Source: CAD feature listing. Evaluate the final solid. Frame: model axes, mm. A direction names the side the tool comes from. Give positions to 0.01 mm unless a question says otherwise; leave off trailing zeros. Write each loop counter-clockwise with the first axis right and the second up, starting at its lowest first coordinate (ties: lowest second). Pieces come first, ordered by that corner, then holes. Notation, with made-up numbers: (61, 76) -> (69, 76) arc R33 ccw to (69, 108) -> close; hole circle Ø5 at (-15.75, 75). An arc over 180 degrees is marked (long way). Use one line per item in the form item = value. Start each with the question number.
(1) First-contact query: P1, Ø5, axis at x = 27, z = 207.5, coming from the -Y side; P2, Ø10, axis at x = 14.5, y = 35.5, coming from the -Z side; P3, Ø8, axis at y = 4.5, z = 180, coming from the -X side. Flat tips, straight axial feed; report the tip coordinate or a pass-through.
(2) Material intervals for line 1 along Y through (x, z) = (0, 8.2); line 2 along Z through (x, y) = (-4, -11); line 3 along Z through (x, y) = (49.5, -9.5), sorted ascending. Write a range as from..to.
(3) Set-up query: faces 1 (the face through (-39.017, 35.777, 144.998)), 2 (the face through (1, 1, 10)), 3 (the face through (45.723, 14.399, 317.255)). Return all of +Z, -Z, +X, -X, +Y, -Y with unobstructed straight access to the full face (end or side cutting, diameter ignored); none if empty.
(4) Cut plane B-B, the plane z = 95. Output: boundary loops of the cut face in (x, y), and give its area (3 significant figures).
from build123d import *

# Parameters (mm, degrees)
SKETCH1_R           = 52.936641772
BOSS_EXTRUDE1_DEPTH = 300
FILLET1_R           = 10
SKETCH2_R           = 47.936641772
BOSS_EXTRUDE2_DEPTH = 50
FILLET2_R           = 15
SKETCH3_R           = 43.922720163
CUT_EXTRUDE1_DEPTH  = 10
FILLET3_R           = 5
FILLET4_R           = 4


with BuildPart() as part:
    # Sketch1 → Boss-Extrude1 (new body)
    with BuildSketch(Plane.XY):
        Circle(SKETCH1_R)
    extrude(amount=BOSS_EXTRUDE1_DEPTH)

    # Fillet1
    fillet1_edges = [part.edges().sort_by_distance(p)[0] for p in [
        (-52.936641772, 0, 300),
    ]]
    fillet(fillet1_edges, radius=FILLET1_R)

    # Sketch2 → Boss-Extrude2 (add)
    with BuildSketch(Plane.XY.offset(300)):
        Circle(SKETCH2_R)
    extrude(amount=BOSS_EXTRUDE2_DEPTH)

    # Fillet2
    fillet2_edges = [part.edges().sort_by_distance(p)[0] for p in [
        (-47.936641772, 0, 350),
    ]]
    fillet(fillet2_edges, radius=FILLET2_R)

    # Sketch3 → Cut-Extrude1 (cut)
    with BuildSketch(Plane(origin=(0, 0, 0), x_dir=(-1, 0, 0), z_dir=(0, 0, -1))):
        Circle(SKETCH3_R)
    extrude(amount=-CUT_EXTRUDE1_DEPTH, mode=Mode.SUBTRACT)

    # Fillet3
    fillet3_edges = [part.edges().sort_by_distance(p)[0] for p in [
        (43.922720163, 0, 0),
    ]]
    fillet(fillet3_edges, radius=FILLET3_R)

    # Fillet4
    fillet4_edges = [part.edges().sort_by_distance(p)[0] for p in [
        (-52.936641772, 0, 0),
    ]]
    fillet(fillet4_edges, radius=FILLET4_R)


solid = part.part
Geometry says:
q1.P1 = -46.93
q1.P2 = 10
q1.P3 = -52.93
q2.line_1 = -52.94..-43.92, 43.92..52.94
q2.line_2 = 10..350
q2.line_3 = 0.28..296.65
q3.face_1 = +Z, -Z
q3.face_2 = -Z
q3.face_3 = +Z
q4.outline = circle Ø105.87 at (0, 0)
q4.area = 8,800 mm^2
